Work out the finished part from the listing and answer in its coordinate system (mm). A direction names the side the tool comes from. Give positions to 0.01 mm unless a question says otherwise; leave off trailing zeros. Loops run counter-clockwise (first coordinate to the right, second up) from the corner with the lowest first, then second, coordinate; pieces in that order, holes last. Notation, with made-up numbers: M 81.5,4 L 109.5,4 A15 ccw 109.5,30 Z; hole C 34.25,86 d6. An arc over 180 degrees is marked long. Answer in a Markdown table with one row per item. Add a question column.
from build123d import *

# Parameters (mm, degrees)
HEX_2_DEPTH = 15


with BuildPart() as part:
    # BodySke → BaseBody (revolve)
    with BuildSketch(Plane.XY, mode=Mode.PRIVATE) as basebody_sk:
        Polygon((0, 0), (0, 10.352), (0.951473244, 12), (38, 12), (50, 0), align=None)
    revolve(basebody_sk.sketch.rotate(Axis((-12.7, 0, 0), (1, 0, 0)), 90), axis=Axis((-12.7, 0, 0), (1, 0, 0)))

    # Sketch2 → Hex 2 (cut)
    with BuildSketch(Plane.ZY):
        Polygon((3.464101615, 6), (-3.464101615, 6), (-6.92820323, 0), (-3.464101615, -6), (3.464101615, -6), (6.92820323, 0), align=None)
    extrude(amount=-HEX_2_DEPTH, mode=Mode.SUBTRACT)


solid = part.part
(1) The mould has two halves that part along Z. Classify faces 1 (the face through (46.75, 1.98, -2.58)), 2 (the face through (15, 0, 0)), 3 (the face through (0, 4, 5)): pulls with the +Z half, pulls with the -Z half, needs draft (parallel to the pull), parting line crosses it, or undercut.
(2) Each of these flat-tipped pins is pushed along its axis until it touches: P1, Ø10, axis at y = 8, z = 1.5, coming from the +X side; P2, Ø8, axis at x = 30.5, z = -4, coming from the +Y side; P3, Ø1.5, axis at x = 19, z = -6.5, coming from the +Y side; P4, Ø3, axis at x = 45, z = -4, coming from the -Y side. Where does it stop, or does it pass through?
(3) Section B-B, the plane x = 22.5 is taken. Determine the outline of the cut face in (y, z).
(4) Consider line 1 along Y through (x, z) = (6, 0); line 2 along Z through (x, y) = (38, -0.5); line 3 along X through (y, z) = (0.75, 1.5). Determine where each line is inside the solid, lowest interval first. Write a range as from..to.
(5) Section A-A, the plane x = 12 is taken. Determine the outline of the cut face in (y, z), and give its area (3 significant figures).
(6) Which of the six approach directions +Z, -Z, +X, -X, +Y, -Y give full straight-line access (tool end or side, diameter ignored) to faces 4 (the face through (19.735, -3.604, 11.446)), 5 (the face through (7.4, 2.96, 5.22))?
Numbers:
| question | item | result |
|---|---|---|
| 1 | face 1 | parting line crosses it |
| 1 | face 2 | undercut |
| 1 | face 3 | needs draft |
| 2 | P1 | stops at x = 46.86 |
| 2 | P2 | stops at y = 12 |
| 2 | P3 | stops at y = 10.53 |
| 2 | P4 | stops at y = -5.4 |
| 3 | outline | C 0,0 d24 |
| 4 | line 1 | y = -12..-6, 6..12 |
| 4 | line 2 | z = -11.99..11.99 |
| 4 | line 3 | x = 15..48.32 |
| 5 | outline | C 0,0 d24; hole M -6,-3.46 L 0,-6.93 L 6,-3.46 L 6,3.46 L 0,6.93 L -6,3.46 Z |
| 5 | area | 328 mm² |
| 6 | face 4 | +X, -X |
| 6 | face 5 | -X |
